Read the model definition and answer for the solid it produces. Units are mm, in the model's axes. Face numbers are marked on the shaded views. A direction names the side the tool comes from. Round coordinates to 2 decimals unless told otherwise and drop trailing zeros. Order: outer loops, then holes, each group sorted by start corner. A loop starts at its lowest first (then second) coordinate and runs counter-clockwise, first axis right, second up. Notation, with made-up numbers: (67.25, 32.25) -> (105.25, 32.25) arc R20 cw to (105.25, 45.25) -> close; hole circle Ø4 at (42, -15.75). An arc over 180 degrees is marked (long way). Use a Markdown table: item, result. Add a question column.
1. Consider L1, parallel to Y at x = 6.5, z = 14.25; L2, parallel to X at y = -18, z = 6; L3, parallel to X at y = 2.5, z = 6. Determine where each line is inside the solid, lowest interval first. Write a range as [from, to].
2. For the marked faces 5 and 6, determine the directions among +Z, -Z, +X, -X, +Y, -Y from which every point of the face is accessible in a straight line to the end or side of a thin tool.
3. Section B-B, the plane z = 6.75 is taken. Give the vertices of the cut face in (x, y), then the cut area to 3 significant figures.
4. Section A-A, the plane y = -18.5 is taken. Give the vertices of the cut face in (x, z).
5. Given pin 1 (12 mm diameter, centred on x = 19.5, y = 12, fed in from +Z); pin 2 (6 mm diameter, centred on y = -7.5, z = 7, fed in from +X); pin 3 (4 mm diameter, centred on x = -25.12, y = -29.27, fed in from -Z); pin 4 (4.5 mm diameter, centred on x = 24.88, y = 20.73, fed in from +Z), each flat-ended and moving along its own axis, determine where each tip first touches the part or whether it passes through.
6. The mould has two halves that part along Y. Classify the marked faces 1, 2, 3 and 4: +Y half, -Y half, draft (parallel to the pull), parting line (faces both ways), or undercut.
7. Section D-D, the plane y = -6 is taken. Give the vertices of the cut face in (x, z), then the cut area to 3 significant figures.
8. Section C-C, the plane x = 6.5 is taken. Give the vertices of the cut face in (y, z), then the cut area to 3 significant figures.
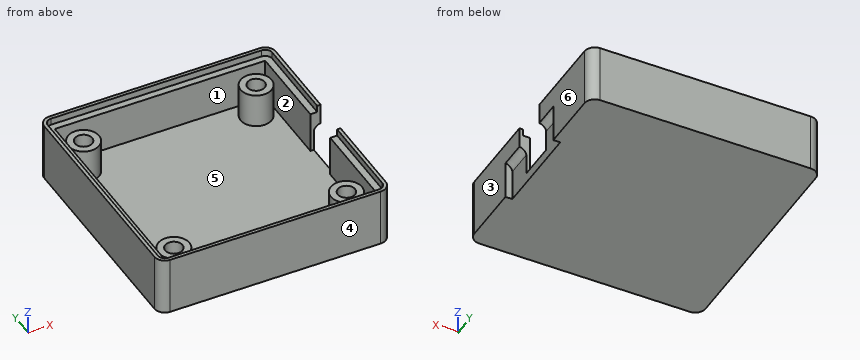
```python
from build123d import *

# Parameters (mm, degrees)
SKETCH1_W           = 67
SKETCH1_H           = 67
BOSS_EXTRUDE1_DEPTH = 17
SKETCH2_W           = 61
SKETCH2_H           = 61
CUT_EXTRUDE1_DEPTH  = 14
CUT_EXTRUDE2_START  = 17
SKETCH3_W           = 65
SKETCH3_H           = 65
CUT_EXTRUDE2_DEPTH  = 2
FILLET1_R           = 3
FILLET3_R           = 2
FILLET4_R           = 2
FILLET5_R           = 2
FILLET6_R           = 2
FILLET7_R           = 3
FILLET8_R           = 3
FILLET9_R           = 3
SKETCH4_R           = 4.5
SKETCH4_R_2         = 2.5
BOSS_EXTRUDE2_DEPTH = 10
SKETCH5_R           = 2.5
BOSS_EXTRUDE3_DEPTH = 5
SKETCH6_W           = 28
SKETCH6_H           = 11
CUT_EXTRUDE3_DEPTH  = 6
SKETCH7_W           = 21.976496756
SKETCH7_H           = 26.513580245
CUT_EXTRUDE4_DEPTH  = 2
FILLET12_SIZE       = 2
FILLET13_SIZE       = 2


with BuildPart() as part:
    # Sketch1 → Boss-Extrude1 (new body)
    with BuildSketch(Plane.XY):
        with Locations((-0.121691543, -4.270311459)):
            Rectangle(SKETCH1_W, SKETCH1_H)
    extrude(amount=BOSS_EXTRUDE1_DEPTH)

    # Sketch2 → Cut-Extrude1 (cut)
    with BuildSketch(Plane.XY.offset(17)):
        with Locations((-0.121691543, -4.270311459)):
            Rectangle(SKETCH2_W, SKETCH2_H)
    extrude(amount=-CUT_EXTRUDE1_DEPTH, mode=Mode.SUBTRACT)

    # Sketch3 → Cut-Extrude2 (cut)
    with BuildSketch(Plane.XY.offset(CUT_EXTRUDE2_START)):
        with Locations((-0.121691543, -4.270311459)):
            Rectangle(SKETCH3_W, SKETCH3_H)
    extrude(amount=-CUT_EXTRUDE2_DEPTH, mode=Mode.SUBTRACT)

    # Fillet1
    fillet1_edges = [part.edges().sort_by_distance(p)[0] for p in [
        (-33.621691543, -37.770311459, 8.5),
    ]]
    fillet(fillet1_edges, radius=FILLET1_R)

    # Fillet3
    fillet3_edges = [part.edges().sort_by_distance(p)[0] for p in [
        (-32.621691543, -36.770311459, 16),
    ]]
    fillet(fillet3_edges, radius=FILLET3_R)

    # Fillet4
    fillet4_edges = [part.edges().sort_by_distance(p)[0] for p in [
        (-32.621691543, 28.229688541, 16),
    ]]
    fillet(fillet4_edges, radius=FILLET4_R)

    # Fillet5
    fillet5_edges = [part.edges().sort_by_distance(p)[0] for p in [
        (32.378308457, 28.229688541, 16),
    ]]
    fillet(fillet5_edges, radius=FILLET5_R)

    # Fillet6
    fillet6_edges = [part.edges().sort_by_distance(p)[0] for p in [
        (32.378308457, -36.770311459, 16),
    ]]
    fillet(fillet6_edges, radius=FILLET6_R)

    # Fillet7
    fillet7_edges = [part.edges().sort_by_distance(p)[0] for p in [
        (33.378308457, -37.770311459, 8.5),
    ]]
    fillet(fillet7_edges, radius=FILLET7_R)

    # Fillet8
    fillet8_edges = [part.edges().sort_by_distance(p)[0] for p in [
        (33.378308457, 29.229688541, 8.5),
    ]]
    fillet(fillet8_edges, radius=FILLET8_R)

    # Fillet9
    fillet9_edges = [part.edges().sort_by_distance(p)[0] for p in [
        (-33.621691543, 29.229688541, 8.5),
    ]]
    fillet(fillet9_edges, radius=FILLET9_R)

    # Sketch4 → Boss-Extrude2 (add)
    # profile 1 of 4: a face of its own
    with BuildSketch(Plane.XY.offset(3)):
        with Locations(Location((24.878308457, -29.270311459, 0), (0, 0, 180))):
            Circle(SKETCH4_R)
        with Locations((24.878308457, -29.270311459)):
            Circle(SKETCH4_R_2, mode=Mode.SUBTRACT)
    # profile 2 of 4: a face of its own
    with BuildSketch(Plane.XY.offset(3)):
        with Locations(Location((-25.121691543, -29.270311459, 0), (0, 0, 180))):
            Circle(SKETCH4_R)
        with Locations((-25.121691543, -29.270311459)):
            Circle(SKETCH4_R_2, mode=Mode.SUBTRACT)
    # profile 3 of 4: a face of its own
    with BuildSketch(Plane.XY.offset(3)):
        with Locations(Location((-25.121691543, 20.729688541, 0), (0, 0, 180))):
            Circle(SKETCH4_R)
        with Locations((-25.121691543, 20.729688541)):
            Circle(SKETCH4_R_2, mode=Mode.SUBTRACT)
    # profile 4 of 4: a face of its own
    with BuildSketch(Plane.XY.offset(3)):
        with Locations(Location((24.878308457, 20.729688541, 0), (0, 0, 180))):
            Circle(SKETCH4_R)
        with Locations((24.878308457, 20.729688541)):
            Circle(SKETCH4_R_2, mode=Mode.SUBTRACT)
    extrude(amount=BOSS_EXTRUDE2_DEPTH)

    # Sketch5 → Boss-Extrude3 (add)
    with BuildSketch(Plane.XY.offset(3)):
        with Locations((24.878308457, -29.270311459)):
            Circle(SKETCH5_R)
        with Locations((-25.121691543, -29.270311459)):
            Circle(SKETCH5_R)
        with Locations((-25.121691543, 20.729688541)):
            Circle(SKETCH5_R)
        with Locations((24.878308457, 20.729688541)):
            Circle(SKETCH5_R)
    extrude(amount=BOSS_EXTRUDE3_DEPTH)

    # Sketch6 → Cut-Extrude3 (cut)
    with BuildSketch(Plane(origin=(33.378308457, 0, 0), x_dir=(0, 0, -1), z_dir=(1, 0, 0))):
        with Locations((-17, -4.270311459)):
            Rectangle(SKETCH6_W, SKETCH6_H)
    extrude(amount=-CUT_EXTRUDE3_DEPTH, mode=Mode.SUBTRACT)

    # Sketch7 → Cut-Extrude4 (cut)
    with BuildSketch(Plane(origin=(33.378308457, 0, 0), x_dir=(0, 0, -1), z_dir=(1, 0, 0))):
        with Locations((0, -4.27031146)):
            Rectangle(SKETCH7_W, SKETCH7_H)
    extrude(amount=-CUT_EXTRUDE4_DEPTH, mode=Mode.SUBTRACT)

    # Fillet12
    # a fillet whose section is not a circle: 2 mm, written as the material it adds along each edge
    with BuildSketch(Plane(origin=(31.378308457, 1.229688541, 10.988248378), x_dir=(0, 0, -1), z_dir=(0, 1, 0))) as fillet12_piece_1:
        with BuildLine():
            Bezier((FILLET12_SIZE, 0), (0, 0), (0, -FILLET12_SIZE), weights=[1, 0.471404521, 1])
            Line((0, -FILLET12_SIZE), (0, 0))
            Line((0, 0), (FILLET12_SIZE, 0))
        make_face()
    extrude(amount=12.756790123)

    # Fillet13
    # a fillet whose section is not a circle: 2 mm, written as the material it adds along each edge
    with BuildSketch(Plane(origin=(31.378308457, -22.527101582, 10.988248378), x_dir=(0, 0, -1), z_dir=(0, 1, 0))) as fillet13_piece_1:
        with BuildLine():
            Bezier((FILLET13_SIZE, 0), (0, 0), (0, -FILLET13_SIZE), weights=[1, 0.471404521, 1])
            Line((0, -FILLET13_SIZE), (0, 0))
            Line((0, 0), (FILLET13_SIZE, 0))
        make_face()
    extrude(amount=12.756790123)


solid = part.part
```
Verdict:
| question | item | result |
|---|---|---|
| 1 | L1 | y = [-37.77, -34.77], [26.23, 29.23] |
| 1 | L2 | x = [-33.62, -30.62], [30.38, 33.38] |
| 1 | L3 | x = [-33.62, -30.62], [30.38, 31.38] |
| 2 | face 5 | +Z |
| 2 | face 6 | +Z, -Z, +X, +Y, -Y |
| 3 | outline | (-33.62, -34.77) arc R3 ccw to (-30.62, -37.77) -> (30.38, -37.77) arc R3 ccw to (33.38, -34.77) -> (33.38, -17.53) -> (31.38, -17.53) -> (31.38, -9.77) -> (30.38, -9.77) -> (30.38, -34.77) -> (-30.62, -34.77) -> (-30.62, 26.23) -> (30.38, 26.23) -> (30.38, 1.23) -> (31.38, 1.23) -> (31.38, 8.99) -> (33.38, 8.99) -> (33.38, 26.23) arc R3 ccw to (30.38, 29.23) -> (-30.62, 29.23) arc R3 ccw to (-33.62, 26.23) -> close; circle Ø9 at (-25.12, -29.27); circle Ø9 at (-25.12, 20.73); circle Ø9 at (24.88, -29.27); circle Ø9 at (24.88, 20.73) |
| 3 | area | 951 mm2 |
| 4 | outline | (-33.62, 0) -> (33.38, 0) -> (33.38, 17) -> (32.38, 17) -> (32.38, 15) -> (30.38, 15) -> (30.38, 3) -> (-30.62, 3) -> (-30.62, 15) -> (-32.62, 15) -> (-32.62, 17) -> (-33.62, 17) -> close |
| 5 | pin 1 | stops at z = 13 |
| 5 | pin 2 | stops at x = 31.38 |
| 5 | pin 3 | stops at z = 0 |
| 5 | pin 4 | stops at z = 8 |
| 6 | face 1 | undercut |
| 6 | face 2 | undercut |
| 6 | face 3 | draft |
| 6 | face 4 | -Y half |
| 7 | outline | (-33.62, 0) -> (31.38, 0) -> (31.38, 3) -> (-30.62, 3) -> (-30.62, 15) -> (-32.62, 15) -> (-32.62, 17) -> (-33.62, 17) -> close |
| 7 | area | 233 mm2 |
| 8 | outline | (-37.77, 0) -> (29.23, 0) -> (29.23, 17) -> (28.23, 17) -> (28.23, 15) -> (26.23, 15) -> (26.23, 3) -> (-34.77, 3) -> (-34.77, 15) -> (-36.77, 15) -> (-36.77, 17) -> (-37.77, 17) -> close |
| 8 | area | 277 mm2 |
